```python
from build123d import *

# Parameters (mm, degrees)
BOSS_EXTRUDE1_DEPTH  = 1.5
SKETCH1_8_R          = 4.1
BOSS_EXTRUDE3_DEPTH  = 36
SKETCH1_9_R          = 5.05
BOSS_EXTRUDE4_DEPTH  = 19
SHELL1_START         = 2
SHELL1_OUTLINE_R     = 2.1
SHELL1_DEPTH         = 32
SHELL1_2_OUTLINE_R   = 3.05
SHELL1_2_OUTLINE_R_2 = 2.1
SHELL1_2_DEPTH       = 15
SKETCH1_10_R         = 3.25
CUT_EXTRUDE1_DEPTH   = 17
SKETCH1_3_R          = 3.25
BOSS_EXTRUDE2_DEPTH  = 6
CHAMFER1_SIZE        = 2
CHAMFER1_SIZE2       = 0.727940469
CHAMFER2_SIZE        = 2.747477419
CHAMFER2_SIZE_2      = 1
CHAMFER3_SIZE        = 1.212435565
CHAMFER3_SIZE_2      = 0.7
CHAMFER6_SIZE        = 0.3
FILLET1_R            = 3.2
CHAMFER5_SIZE        = 0.3
FILLET2_R            = 1
FILLET3_R            = 2


# Read off the part's stored shape, not the designer's step: Shell1
with BuildPart() as part:
    # Sketch1 → Boss-Extrude1 (new body)
    with BuildSketch(Plane.XY):
        Polygon((-11.2, 6.466323015), (0, 12.93264603), (11.2, 6.466323015), (11.2, -6.466323015), (0, -12.93264603), (-11.2, -6.466323015), align=None)
    extrude(amount=BOSS_EXTRUDE1_DEPTH)

    # Sketch1<8> → Boss-Extrude3 (add)
    with BuildSketch(Plane.XY):
        with Locations(Location((0, 0, 0), (0, 0, 180))):
            Circle(SKETCH1_8_R)
    extrude(amount=BOSS_EXTRUDE3_DEPTH)

    # Sketch1<9> → Boss-Extrude4 (add)
    with BuildSketch(Plane.XY):
        with Locations(Location((0, 0, 0), (0, 0, 180))):
            Circle(SKETCH1_9_R)
    extrude(amount=BOSS_EXTRUDE4_DEPTH)

    # Shell1 outline → Shell1 (cut)
    with BuildSketch(Plane.XY.offset(SHELL1_START)):
        Circle(SHELL1_OUTLINE_R)
    extrude(amount=SHELL1_DEPTH, mode=Mode.SUBTRACT)

    # Shell1 2 outline → Shell1 2 (cut)
    with BuildSketch(Plane.XY.offset(SHELL1_START)):
        Circle(SHELL1_2_OUTLINE_R)
        Circle(SHELL1_2_OUTLINE_R_2, mode=Mode.SUBTRACT)
    extrude(amount=SHELL1_2_DEPTH, mode=Mode.SUBTRACT)

    # Sketch1<10> → Cut-Extrude1 (cut)
    with BuildSketch(Plane.XY):
        Circle(SKETCH1_10_R)
    extrude(amount=CUT_EXTRUDE1_DEPTH, mode=Mode.SUBTRACT)

    # Sketch1<3> → Boss-Extrude2 (add)
    with BuildSketch(Plane.XY):
        Polygon((0, 11.893415545), (10.3, 5.946707773), (10.3, -5.946707773), (0, -11.893415545), (-10.3, -5.946707773), (-10.3, 5.946707773), align=None)
        Circle(SKETCH1_3_R, mode=Mode.SUBTRACT)
    extrude(amount=BOSS_EXTRUDE2_DEPTH)

    # Chamfer1
    chamfer1_edges = [part.edges().sort_by_distance(p)[0] for p in [
        (4.1, 0, 36),
    ]]
    chamfer1_side = [part.faces().sort_by_distance(p)[0] for p in [
        (4.1, 0, 27.5),
    ]]
    chamfer(chamfer1_edges, length=CHAMFER1_SIZE, length2=CHAMFER1_SIZE2, reference=chamfer1_side[0])

    # Chamfer2
    # the kernel refuses this chamfer: 2.747477419, 1 mm, written as the material it adds along each edge
    with BuildSketch(Plane(origin=(0, 0, 19), x_dir=(-1, 0, 0), z_dir=(0, -1, 0))) as chamfer2_piece_1_section:
        Polygon((4.1, -CHAMFER2_SIZE), (4.1 + CHAMFER2_SIZE_2, 0), (4.1, 0), align=None)
    chamfer2_piece_1 = revolve(axis=Axis((0, 0, 19), (0, 0, -1)), mode=Mode.PRIVATE)
    chamfer2_piece_1 = chamfer2_piece_1 & Plane(origin=(0, 0, 20.481947897), x_dir=(-1, 0, 0), z_dir=(0, 0, -1)) * Cylinder(5.05, 21, mode=Mode.PRIVATE)
    add(chamfer2_piece_1)

    # Chamfer3
    # the kernel refuses this chamfer: 1.212435565, 0.7 mm, written as the material it takes off along each edge
    with BuildSketch(Plane(origin=(0, 0, 17), x_dir=(1, 0, 0), z_dir=(0, -1, 0))) as chamfer3_piece_1_section:
        Polygon((2.1 + CHAMFER3_SIZE, 0), (2.1, CHAMFER3_SIZE_2), (2.1, 0), align=None)
    chamfer3_piece_1 = revolve(axis=Axis((0, 0, 17), (0, 0, 1)), mode=Mode.PRIVATE)
    chamfer3_piece_1 = chamfer3_piece_1 & Plane(origin=(0, 0, 17.363214185), x_dir=(1, 0, 0), z_dir=(0, 0, -1)) * Cylinder(3.25, 14, mode=Mode.PRIVATE)
    add(chamfer3_piece_1, mode=Mode.SUBTRACT)

    # Chamfer6
    chamfer6_edges = [part.edges().sort_by_distance(p)[0] for p in [
        (-3.25, 0, 0),
    ]]
    chamfer(chamfer6_edges, length=CHAMFER6_SIZE)

    # Fillet1
    fillet1_edges = [part.edges().sort_by_distance(p)[0] for p in [
        (-10.3, -5.946707773, 3.75),
        (0, -11.893415545, 3.75),
        (10.3, -5.946707773, 3.75),
        (10.3, 5.946707773, 3.75),
        (0, 11.893415545, 3.75),
        (-10.3, 5.946707773, 3.75),
    ]]
    fillet(fillet1_edges, radius=FILLET1_R)

    # Chamfer5
    chamfer5_edges = [part.edges().sort_by_distance(p)[0] for p in [
        (-5.15, -8.920061659, 6),
        (5.15, 8.920061659, 6),
        (-5.15, 8.920061659, 6),
        (-10.3, 0, 6),
        (9.871281292, 5.699186911, 6),
        (0, 11.398373822, 6),
        (-9.871281292, 5.699186911, 6),
        (-9.871281292, -5.699186911, 6),
        (0, -11.398373822, 6),
        (9.871281292, -5.699186911, 6),
        (5.6, 9.699484522, 1.5),
        (11.2, 0, 1.5),
        (5.6, -9.699484522, 1.5),
        (-5.6, -9.699484522, 1.5),
        (-11.2, 0, 1.5),
        (-5.6, 9.699484522, 1.5),
        (10.3, 0, 6),
        (5.15, -8.920061659, 6),
    ]]
    chamfer(chamfer5_edges, length=CHAMFER5_SIZE)

    # Fillet2
    fillet2_edges = [part.edges().sort_by_distance(p)[0] for p in [
        (11.2, 6.466323015, 0.6),
        (11.2, -6.466323015, 0.6),
        (0, -12.93264603, 0.6),
        (-11.2, -6.466323015, 0.6),
        (-11.2, 6.466323015, 0.6),
        (0, 12.93264603, 0.6),
    ]]
    fillet(fillet2_edges, radius=FILLET2_R)

    # Fillet3
    fillet3_edges = [part.edges().sort_by_distance(p)[0] for p in [
        (5.05, 0, 6),
    ]]
    fillet(fillet3_edges, radius=FILLET3_R)


solid = part.part
```
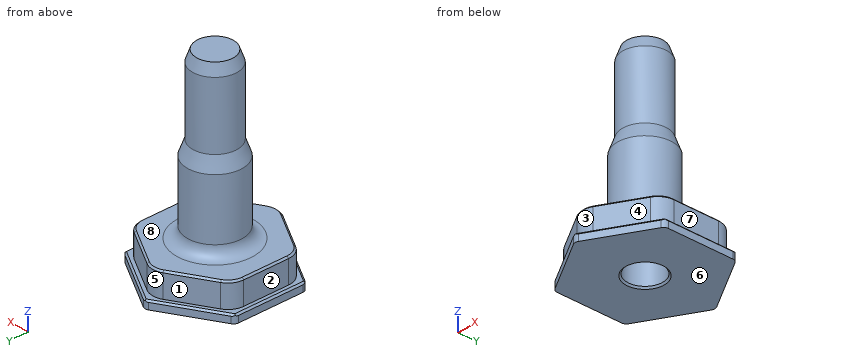
Could you check a few things on this model? Use its own coordinates, in mm. Face numbers are marked on the shaded views. A direction names the side the tool comes from. Coordinates: 2 decimals unless noted, no trailing zeros. Loops run counter-clockwise (first coordinate to the right, second up) from the corner with the lowest first, then second, coordinate; pieces in that order, holes last. Notation, with made-up numbers: M 82.25,-4.75 L 126.25,-4.75 A33 cw 126.25,26.25 Z; hole C 77.25,30 d6. An arc over 180 degrees is marked long. Put each result on its own line as item: value. Start each with the question number.
(1) Suppose I cut it at D-D on z = 26.5. Please give me the cut outline in (x, y), then the cut area to 3 significant figures.
(2) Will these pins go through, and if not, where does the flat tip stop? P1, Ø2.5, axis at x = 0, y = 0, coming from the -Z side; P2, Ø1.3, axis at y = 1, z = 3.5, coming from the +X side; P3, Ø8, axis at x = -6, z = 21.5, coming from the +Y side.
(3) I need wall thicknesses on line 1 (Y direction, x = 0, z = 17); line 2 (Z direction, x = 1.5, y = 10.5); line 3 (X direction, y = 2, z = 8). Which ranges of each line are inside material? Lowest first, please. Write a range as from..to.
(4) Suppose I cut it at A-A on z = 2. Please give me the cut outline in (x, y), then the cut area to 3 significant figures.
(5) Thinking about a two-plate mould opening in Z: for the marked faces 6, 7 and 8, which applies, pulls with the +Z half, pulls with the -Z half, needs draft (parallel to the pull), parting line crosses it, or undercut?
(6) For the marked faces 1, 2, 3, 4 and 5, which set-ups out of +Z, -Z, +X, -X, +Y, -Y let a thin tool reach every point of the face, with its end or its side?
(7) Suppose I cut it at C-C on z = 14.5. Please give me the cut outline in (x, y).
Solutions:
1. outline: C 0,0 d8.2; hole C 0,0 d4.2
1. area: 39.0 mm2
2. P1: stops at z = 34
2. P2: stops at x = 10.3
2. P3: stops at y = 4.22
3. line 1: y = -5.05..-3.25, 3.25..5.05
3. line 2: z = 0..6
3. line 3: x = -4.64..-2.56, 2.56..4.64
4. outline: M -10.3,-4.1 A3.2 ccw -8.7,-6.87 L -1.6,-10.97 A3.2 ccw 1.6,-10.97 L 8.7,-6.87 A3.2 ccw 10.3,-4.1 L 10.3,4.1 A3.2 ccw 8.7,6.87 L 1.6,10.97 A3.2 ccw -1.6,10.97 L -8.7,6.87 A3.2 ccw -10.3,4.1 Z; hole C 0,0 d6.5
4. area: 331 mm2
5. face 6: pulls with the -Z half
5. face 7: needs draft
5. face 8: pulls with the +Z half
6. face 1: +Z, -X, +Y
6. face 2: +Z, -X, +Y, -Y
6. face 3: +Z, -Y
6. face 4: +Z, +X, -Y
6. face 5: +Z, +Y
7. outline: C 0,0 d10.1; hole C 0,0 d6.5
